For this review, take the finished solid that the model builds, in its own axes (mm). Face numbers are marked on the shaded views. A direction names the side the tool comes from. Round coordinates to 2 decimals unless told otherwise and drop trailing zeros. Order: outer loops, then holes, each group sorted by start corner. A loop starts at its lowest first (then second) coordinate and runs counter-clockwise, first axis right, second up. Notation, with made-up numbers: (49.25, 37) -> (90.25, 37) arc R14 cw to (90.25, 63) -> close; hole circle Ø8 at (-21.5, 25.5). An arc over 180 degrees is marked (long way). Answer in a Markdown table with one row per item.
Autodesk Inventor part; units mm, degrees
ref_plane "YZ Plane" through (0, 0, 0) normal (1, 0, 0) x (0, 1, 0)
ref_plane "XZ Plane" through (0, 0, 0) normal (0, 1, 0) x (-1, 0, 0)
ref_plane "XY Plane" through (0, 0, 0) normal (0, 0, 1) x (1, 0, 0)
sketch "Sketch1" plane through (0, 0, 0) normal (0, 1, 0) x (-1, 0, 0)
  line L0 (0, -88.9) -> (0, 88.9)
  line L1 (-26.67, 0) -> (26.67, 0)
  line L2 (26.67, 0) -> (-26.67, 0)
  line L3 (0, -88.9) -> (0, 88.9)
  line L4 (19.05, 63.5) -> (-19.05, 63.5)
  line L5 (-19.05, 63.5) -> (-19.05, -63.5)
  line L6 (-19.05, -63.5) -> (19.05, -63.5)
  line L7 (19.05, -63.5) -> (19.05, 63.5)
  line L8 (19.05, 63.5) -> (-19.05, -63.5) construction
  line L9 (-19.05, 63.5) -> (19.05, -63.5) construction
  point P0 (0, 0)
  dimension "d0" = 38.1
  dimension "d1" = 127
extrude "Extrusion1" add sketch "Sketch1" along normal blind 177.8
sketch "Sketch2" plane through (0, 0, 0) normal (0, -1, 0) x (1, 0, 0)
  line L0 (-25.4, -63.5) -> (25.4, -63.5)
  line L1 (25.4, -63.5) -> (25.4, 63.5)
  line L2 (25.4, 63.5) -> (-25.4, 63.5)
  line L3 (-25.4, 63.5) -> (-25.4, -63.5)
  line L4 (-25.4, -63.5) -> (25.4, 63.5) construction
  line L5 (25.4, -63.5) -> (-25.4, 63.5) construction
  point P0 (0, 0)
  dimension "d4" = 50.8
extrude "Extrusion2" add sketch "Sketch2" against normal blind 3.81
properties part number "Netgear Router" material "Acetal Resin, Black"
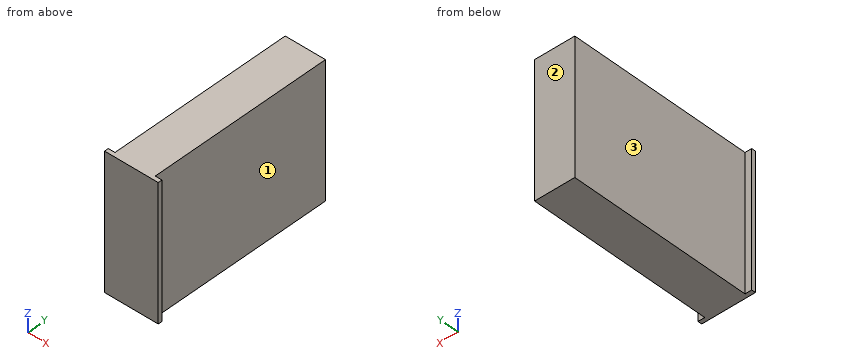
Q1. Take a section at B-B, the plane y = 70. Write out the cut boundary in (x, z), then the cut area to 3 significant figures.
Answer key:
| item | result |
|---|---|
| outline | (-19.05, -63.5) -> (19.05, -63.5) -> (19.05, 63.5) -> (-19.05, 63.5) -> close |
| area | 4,840 mm^2 |
Q2. To check wall thickness, follow probe 1 along X at (y, z) = (19, 51); probe 2 along Y at (x, z) = (-21, 58.5). State the ranges of each line that lie inside material, in increasing order.
Answer key:
| item | result |
|---|---|
| probe 1 | x = -19.05 to 19.05 |
| probe 2 | y = 0 to 3.81 |
Q3. Take a section at A-A, the plane z = 51. Write out the cut boundary in (x, y), then the cut area to 3 significant figures.
Answer key:
| item | result |
|---|---|
| outline | (-25.4, 0) -> (25.4, 0) -> (25.4, 3.81) -> (19.05, 3.81) -> (19.05, 177.8) -> (-19.05, 177.8) -> (-19.05, 3.81) -> (-25.4, 3.81) -> close |
| area | 6,820 mm^2 |
Q4. Tool access review of the marked faces 1, 2 and 3: name each direction out of +Z, -Z, +X, -X, +Y, -Y from which nothing blocks a thin tool from reaching the whole face with its end or side.
Answer key:
| item | result |
|---|---|
| face 1 | +Z, -Z, +X, +Y |
| face 2 | +Z, -Z, +X, -X, +Y |
| face 3 | +Z, -Z, -X, +Y |
Q5. Take a section at C-C, the plane x = -21. Write out the cut boundary in (y, z), then the cut area to 3 significant figures.
Answer key:
| item | result |
|---|---|
| outline | (0, -63.5) -> (3.81, -63.5) -> (3.81, 63.5) -> (0, 63.5) -> close |
| area | 484 mm^2 |
Q6. Clearance check with a flat-ended pin moving along its axis: pin 1 Ø3 at (y, z) = (126, 23.5) entering from -X. State where the tip first meets the part, or that it passes through.
Answer key:
| item | result |
|---|---|
| pin 1 | stops at x = -19.05 |
